Verification items for the finished model (mm, model axes). A direction names the side the tool comes from. Coordinates: 2 decimals unless noted, no trailing zeros. Loops run counter-clockwise (first coordinate to the right, second up) from the corner with the lowest first, then second, coordinate; pieces in that order, holes last. Notation, with made-up numbers: (-15.75, 51.5) - (3.25, 51.5) arc R20 ccw to (3.25, 81.5) - close; hole circle Ø5 at (75, -3.75). An arc over 180 degrees is marked (long way). One line per item, written item: value. Start each with the question number.
(1) Set-up check for faces 1 (the face through (-21.2, 0, 1)), 2 (the face through (0, 0, 3)), 3 (the face through (-3.8, -14, 1)), 4 (the face through (-20.7, 0, 2)), 5 (the face through (20.7, 0, 2)): record each of +Z, -Z, +X, -X, +Y, -Y from which the full face is reachable in a straight line by a thin tool's end or side.
(2) Section check A-A (y = -10.5). Record the boundary of the cut face in (x, z).
(3) Section check B-B (z = 0.5). Record the boundary of the cut face in (x, y), plus the area to 3 significant figures.
(4) Gauge pin test, flat ends, axial feed: P1, Ø0.8, axis at y = -4, z = 2, coming from the +X side; P2, Ø0.8, axis at y = -1, z = 2.5, coming from the -X side. Record the tip position at first contact, or that the pin passes through.
(5) Thickness scan on probe 1 along X at (y, z) = (-12, 0.9); probe 2 along X at (y, z) = (-10.5, 2.65); probe 3 along X at (y, z) = (16, 2). Record the ranges inside material, lowest first. Write a range as [from, to].
(6) Section check C-C (x = -1). Record the boundary of the cut face in (y, z), plus the area to 3 significant figures.
```python
from build123d import *

# Parameters (mm, degrees)
SKETCH1_W           = 42.4
SKETCH1_H           = 37
BOSS_EXTRUDE1_DEPTH = 1.5
SKETCH2_W           = 41.4
SKETCH2_H           = 37
BOSS_EXTRUDE2_DEPTH = 1.5
SKETCH3_W           = 11.6
SKETCH3_H           = 10
CUT_EXTRUDE1_DEPTH  = 29.29646621
FILLET1_R           = 1


with BuildPart() as part:
    # Sketch1 → Boss-Extrude1 (new body)
    with BuildSketch(Plane.XY):
        Rectangle(SKETCH1_W, SKETCH1_H)
    extrude(amount=BOSS_EXTRUDE1_DEPTH)

    # Sketch2 → Boss-Extrude2 (add)
    with BuildSketch(Plane.XY.offset(1.5)):
        Rectangle(SKETCH2_W, SKETCH2_H)
    extrude(amount=BOSS_EXTRUDE2_DEPTH)

    # Sketch3 → Cut-Extrude1 (cut, through all)
    with BuildSketch(Plane(origin=(0, 0, 0), x_dir=(-1, 0, 0), z_dir=(0, 0, -1))):
        with Locations((-2, -13.5)):
            Rectangle(SKETCH3_W, SKETCH3_H)
    extrude(amount=-CUT_EXTRUDE1_DEPTH, mode=Mode.SUBTRACT)

    # Fillet1
    fillet1_edges = [part.edges().sort_by_distance(p)[0] for p in [
        (7.8, -8.5, 1.5),
        (-3.8, -8.5, 1.5),
    ]]
    fillet(fillet1_edges, radius=FILLET1_R)


solid = part.part
```
Responses:
1. face 1: +Z, -Z, -X, +Y, -Y
1. face 2: +Z, +X, -X, +Y, -Y
1. face 3: +Z, -Z, -Y
1. face 4: +Z, -X, +Y, -Y
1. face 5: +Z, +X, +Y, -Y
2. outline: (-21.2, 0) - (-3.8, 0) - (-3.8, 3) - (-20.7, 3) - (-20.7, 1.5) - (-21.2, 1.5) - close; (7.8, 0) - (21.2, 0) - (21.2, 1.5) - (20.7, 1.5) - (20.7, 3) - (7.8, 3) - close
3. outline: (-21.2, -18.5) - (-3.8, -18.5) - (-3.8, -9.5) arc R1 cw to (-2.8, -8.5) - (6.8, -8.5) arc R1 cw to (7.8, -9.5) - (7.8, -18.5) - (21.2, -18.5) - (21.2, 18.5) - (-21.2, 18.5) - close
3. area: 1,450 mm²
4. P1: stops at x = 20.7
4. P2: stops at x = -20.7
5. probe 1: x = [-21.2, -3.8], [7.8, 21.2]
5. probe 2: x = [-20.7, -3.8], [7.8, 20.7]
5. probe 3: x = [-20.7, 20.7]
6. outline: (-8.5, 0) - (18.5, 0) - (18.5, 3) - (-8.5, 3) - close
6. area: 81.0 mm²
